```python
from build123d import *

# Parameters (mm, degrees)
SKETCH_R     = 15
PAD_DEPTH    = 10
POCKET_DEPTH = 10


with BuildPart() as part:
    # Sketch → Pad (new body, symmetric)
    with BuildSketch(Plane.YZ):
        Circle(SKETCH_R)
    extrude(amount=PAD_DEPTH, both=True)

    # Sketch001 (on Face3 of Pad) → Pocket (cut)
    with BuildSketch(Plane.YZ.offset(10)):
        with BuildLine():
            Line((3.535534, -3.535534), (7.071068, -7.071068))
            ThreePointArc((-7.071068, -7.071068), (0, -10), (7.071068, -7.071068))
            Line((-3.535534, -3.535534), (-7.071068, -7.071068))
            ThreePointArc((-3.535534, 3.535534), (-5, 0), (-3.535534, -3.535534))
            Line((-3.535534, 3.535534), (-7.071068, 7.071068))
            ThreePointArc((7.071068, 7.071068), (0, 10), (-7.071068, 7.071068))
            Line((3.535534, 3.535534), (7.071068, 7.071068))
            ThreePointArc((3.535534, -3.535534), (5, 0), (3.535534, 3.535534))
        make_face()
    extrude(amount=-POCKET_DEPTH, mode=Mode.SUBTRACT)


solid = part.part
```
Geometry check sheet. Reference: the model listing, model coordinates, mm. A direction names the side the tool comes from. Round coordinates to 2 decimals unless told otherwise and drop trailing zeros. Loops run counter-clockwise (first coordinate to the right, second up) from the corner with the lowest first, then second, coordinate; pieces in that order, holes last. Notation, with made-up numbers: (56, 49) - (104, 49) arc R28 cw to (104, 71) - close; hole circle Ø2 at (-23.75, 24.5). An arc over 180 degrees is marked (long way). Use a Markdown table: item, result.
Q1. Cross-section at A-A on z = 0. Record the cut outline in (x, y).
Solutions:
| item | result |
|---|---|
| outline | (-10, -15) - (10, -15) - (10, -5) - (0, -5) - (0, 5) - (10, 5) - (10, 15) - (-10, 15) - close |
Q2. Cross-section at B-B on y = 0. Record the cut outline in (x, z).
Solutions:
| item | result |
|---|---|
| outline | (-10, -15) - (10, -15) - (10, -10) - (0, -10) - (0, 10) - (10, 10) - (10, 15) - (-10, 15) - close |
Q3. Draft check along Y on faces 1 (the flat face through (-10, 0, 0)), 2 (the cylindrical face through (0.14, -14.985, 0.66)), 3 (the cylindrical face through (5, -5, 0)). Enter one of: released by +Y, released by -Y, zero draft, split by the parting line, or undercut.
Solutions:
| item | result |
|---|---|
| face 1 | zero draft |
| face 2 | split by the parting line |
| face 3 | undercut |
Q4. Access from +Z, -Z, +X, -X, +Y, -Y to the whole of each face (thin tool, end or side, straight path). Record for faces 4 (the flat face through (5, -5, 5)), 5 (the flat face through (10, 6, 0)).
Solutions:
| item | result |
|---|---|
| face 4 | +X |
| face 5 | +Z, -Z, +X, +Y, -Y |
Q5. Cross-section at D-D on y = 5.5. Record the cut outline in (x, z).
Solutions:
| item | result |
|---|---|
| outline | (-10, -13.96) - (10, -13.96) - (10, -8.35) - (0, -8.35) - (0, -5.5) - (10, -5.5) - (10, 5.5) - (0, 5.5) - (0, 8.35) - (10, 8.35) - (10, 13.96) - (-10, 13.96) - close |
Q6. Go/stop test with flat-tipped pins: P1, Ø4, axis at x = 2.5, z = -3.5, coming from the -Y side; P2, Ø12, axis at x = -2.5, y = -11.5, coming from the -Z side; P3, Ø1, axis at x = -6, y = -4.5, coming from the +Z side. Record where each tip stops, or that it passes through.
Solutions:
| item | result |
|---|---|
| P1 | stops at y = -14.92 |
| P2 | stops at z = -13.96 |
| P3 | stops at z = 14.46 |
Q7. Cross-section at C-C on x = -2.75. Record the cut outline in (y, z), plus the area to 3 significant figures.
Solutions:
| item | result |
|---|---|
| outline | circle Ø30 at (0, 0) |
| area | 707 mm2 |
Q8. Material ranges on line 1 (X direction, y = -0.5, z = 6.5); line 2 (Z direction, x = 2.25, y = -3.25); line 3 (Z direction, x = 3.5, y = 2.5), recorded low to high.
Solutions:
| item | result |
|---|---|
| line 1 | x = -10 to 0 |
| line 2 | z = -14.64 to -9.46, 9.46 to 14.64 |
| line 3 | z = -14.79 to -9.68, 9.68 to 14.79 |
